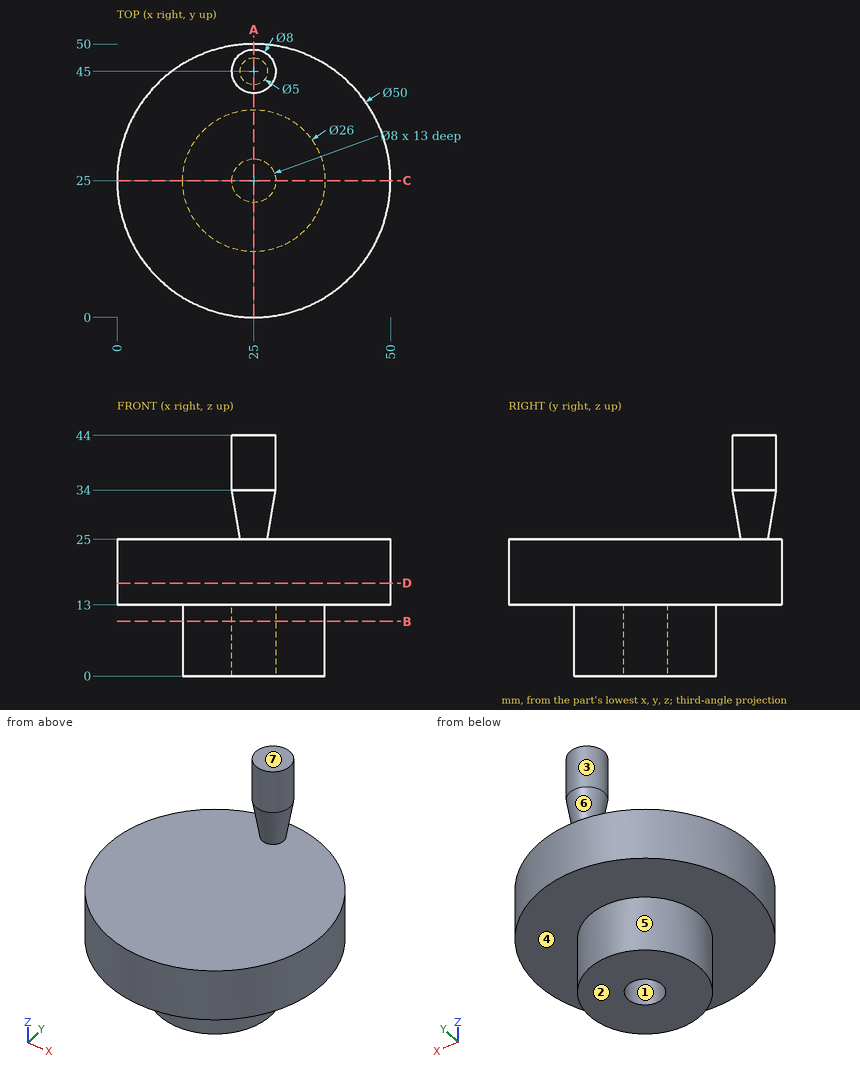
Design review of the part shown in the three views and the two pictorial views. Dimensions are in mm from the part's minimum x, y and z. A direction names the side the tool comes from. Round coordinates to 2 decimals unless told otherwise and drop trailing zeros. Write each loop counter-clockwise with the first axis right and the second up, starting at its lowest first coordinate (ties: lowest second). Pieces come first, ordered by that corner, then holes.
1) Mouldability with a two-part tool opening along Z and no side actions: class the marked faces 4, 5, 6 and 7 as +Z half, -Z half, draft (parallel to the pull), parting line (faces both ways), or undercut.
Answer below:
face 4: -Z half
face 5: draft
face 6: undercut
face 7: +Z half
2) Take a section at D-D on z = 17. Give the boundary of the cut face in (x, y).
Answer below:
outline: circle Ø50 at (25, 25)
3) Machinability: for the marked faces 1, 2 and 3, which of the approach directions +Z, -Z, +X, -X, +Y, -Y give a long, thin tool a straight path to every point of the face, cutting with its end or side? Answer none if there is none.
Answer below:
face 1: -Z
face 2: -Z, +X, -X, +Y, -Y
face 3: +Z
4) Take a section at A-A on x = 25. Give the boundary of the cut face in (y, z).
Answer below:
outline: (0, 13) - (12, 13) - (12, 0) - (21, 0) - (21, 13) - (29, 13) - (29, 0) - (38, 0) - (38, 13) - (50, 13) - (50, 25) - (47.5, 25) - (49, 34) - (49, 44) - (41, 44) - (41, 34) - (42.5, 25) - (0, 25) - close
5) Take a section at B-B on z = 10. Give the boundary of the cut face in (x, y), then the cut area to 3 significant figures.
Answer below:
outline: circle Ø26 at (25, 25); hole circle Ø8 at (25, 25)
area: 481 mm2
6) Insertion check: pin 1 Ø15 at (x, y) = (22, 20.5) entering from +Z; pin 2 Ø12 at (x, z) = (17.5, 5.5) entering from -Y; pin 3 Ø5 at (y, z) = (39.5, 24) entering from -X. Each pin has a flat end and moves straight along its axis. Give the tip position at first contact, or say it passes through.
Answer below:
pin 1: stops at z = 25
pin 2: stops at y = 12.09
pin 3: stops at x = 3.07
7) For line 1 along Y through (x, z) = (25, 9.5); line 2 along Z through (x, y) = (38, 24); line 3 along X through (y, z) = (22, 10.5), list the stretches that pass through material, from the lowest coordinate up.
Answer below:
line 1: y = 12 to 21, 29 to 38
line 2: z = 13 to 25
line 3: x = 12.35 to 22.35, 27.65 to 37.65
8) Take a section at C-C on y = 25. Give the boundary of the cut face in (x, z).
Answer below:
outline: (0, 13) - (12, 13) - (12, 0) - (21, 0) - (21, 13) - (29, 13) - (29, 0) - (38, 0) - (38, 13) - (50, 13) - (50, 25) - (0, 25) - close
